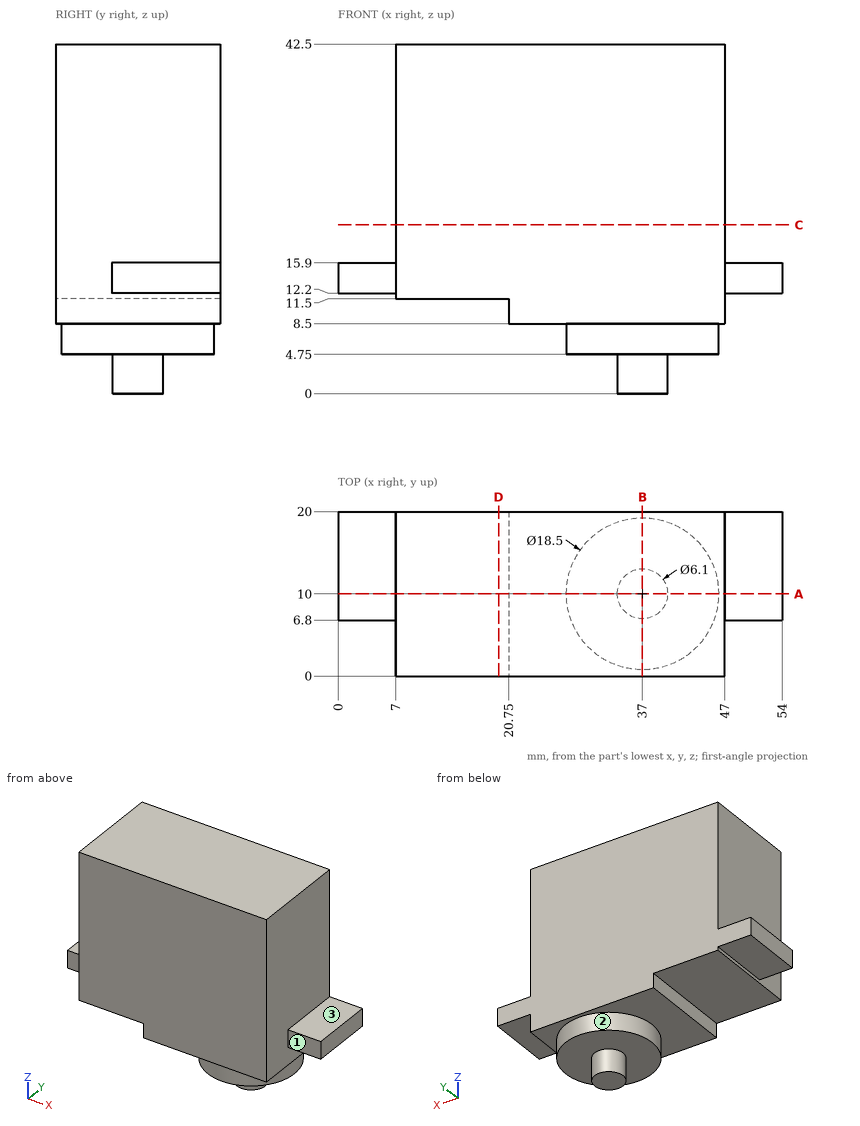
Can you work these out from the drawing? Everything is in mm from the part's minimum corner. A direction names the side the tool comes from. Coordinates: 2 decimals unless noted, no trailing zeros. Loops run counter-clockwise (first coordinate to the right, second up) from the corner with the lowest first, then second, coordinate; pieces in that order, holes last.
1. Imagine slicing it at A-A, the plane y = 10. Please give me the cut outline in (x, z).
2. Imagine slicing it at D-D, the plane x = 19.5. Please give me the cut outline in (y, z).
3. For the marked faces 1, 2 and 3, which set-ups out of +Z, -Z, +X, -X, +Y, -Y let a thin tool reach every point of the face, with its end or its side?
4. For P1, Ø4, axis at y = 14, z = 27, coming from the -X side; P2, Ø7, axis at x = 12, y = 9, coming from the -Z side; P3, Ø3.5, axis at x = 49.5, y = 11, coming from the -Z side, each with a flat end and sliding along its axis, tell me the tip position at first contact or that it passes through.
5. I need wall thicknesses on L1, parallel to Z at x = 9, y = 7; L2, parallel to Z at x = 34.5, y = 19.25; L3, parallel to X at y = 6.25, z = 9. Which ranges of each line are inside material? Lowest first, please.
6. Imagine slicing it at B-B, the plane x = 37. Please give me the cut outline in (y, z), and give its area (3 significant figures).
7. Imagine slicing it at C-C, the plane z = 20.5. Please give me the cut outline in (x, y), and give its area (3 significant figures).
Taken from the geometry:
1. outline: (0, 12.2) - (7, 12.2) - (7, 11.5) - (20.75, 11.5) - (20.75, 8.5) - (27.75, 8.5) - (27.75, 4.75) - (33.95, 4.75) - (33.95, 0) - (40.05, 0) - (40.05, 4.75) - (46.25, 4.75) - (46.25, 8.5) - (47, 8.5) - (47, 12.2) - (54, 12.2) - (54, 15.9) - (47, 15.9) - (47, 42.5) - (7, 42.5) - (7, 15.9) - (0, 15.9) - close
2. outline: (0, 11.5) - (20, 11.5) - (20, 42.5) - (0, 42.5) - close
3. face 1: +Z, -Z, +X, -Y
3. face 2: -Z
3. face 3: +Z, +X, +Y, -Y
4. P1: stops at x = 7
4. P2: stops at z = 11.5
4. P3: stops at z = 12.2
5. L1: z = 11.5 to 42.5
5. L2: z = 8.5 to 42.5
5. L3: x = 20.75 to 47
6. outline: (0, 8.5) - (0.75, 8.5) - (0.75, 4.75) - (6.95, 4.75) - (6.95, 0) - (13.05, 0) - (13.05, 4.75) - (19.25, 4.75) - (19.25, 8.5) - (20, 8.5) - (20, 42.5) - (0, 42.5) - close
6. area: 778 mm2
7. outline: (7, 0) - (47, 0) - (47, 20) - (7, 20) - close
7. area: 800 mm2
